Geometry check sheet. Reference: the model listing, model coordinates, mm. A direction names the side the tool comes from. Give positions to 0.01 mm unless a question says otherwise; leave off trailing zeros. Put each result on its own line as item: value. Start each with the question number.
Q1. Material ranges on L1, parallel to Z at x = 76.2, y = 3.5; L2, parallel to X at y = 2, z = -18 (3 decimals); L3, parallel to X at y = 9.5, z = -101 (3 decimals), recorded low to high.
Q2. Section check A-A on y = 8. State how many separate pieces and enclosed holes the cut face has, then the cut area to 3 significant figures.
Q3. Access from +Z, -Z, +X, -X, +Y, -Y to the whole of each face (thin tool, end or side, straight path). Record for faces 4 (the flat face through (46, 6, 0)), 5 (the flat face through (12.7, 6, -16)).
Q4. Mould release check, pull along X, two halves, no side actions. Record for faces 1 (the cylindrical face through (89.359, 6.439, -136.836)), 2 (the flat face through (85.725, 6, -124)), 3 (the cylindrical face through (2.72, 6.44, -136.84)): +X half, -X half, draft (parallel to the pull), parting line (faces both ways), or undercut.
```python
from build123d import *

# Parameters (mm, degrees)
SKETCH1_W                   = 92.075
SKETCH1_H                   = 139.7
BOSS_EXTRUDE1_DEPTH         = 12.7
F_1_4_0_25_DIAMETER_HOLE1_D = 6.35
CUT_EXTRUDE1_DEPTH          = 12.7
FILLET1_R                   = 9.525


with BuildPart() as part:
    # Sketch1 → Boss-Extrude1 (new body)
    with BuildSketch(Plane(origin=(0, 0, 0), x_dir=(1, 0, 0), z_dir=(0, 1, 0))):
        with Locations((46.0375, 69.85)):
            Rectangle(SKETCH1_W, SKETCH1_H)
    extrude(amount=BOSS_EXTRUDE1_DEPTH)

    # 1/4 (0.25) Diameter Hole1 (through all)
    with Locations(Plane(origin=(0, 12.7, 0), x_dir=(1, 0, 0), z_dir=(0, 1, 0))):
        with Locations((76.2, 36.5125), (46.0375, 69.85), (76.2, 103.1875), (15.875, 36.5125), (15.875, 103.1875)):
            Hole(F_1_4_0_25_DIAMETER_HOLE1_D / 2)

    # Sketch7 → Cut-Extrude1 (cut)
    with BuildSketch(Plane(origin=(0, 12.7, 0), x_dir=(1, 0, 0), z_dir=(0, 1, 0))):
        with BuildLine():
            Line((12.7, 127), (12.7, 120.65))
            ThreePointArc((12.7, 120.65), (9.525, 117.475), (6.35, 120.65))
            Line((6.35, 120.65), (6.35, 127))
            ThreePointArc((6.35, 127), (9.525, 130.175), (12.7, 127))
        make_face()
    cut_extrude1 = extrude(amount=-CUT_EXTRUDE1_DEPTH, mode=Mode.SUBTRACT)

    # Sketch-Pattern1: Cut-Extrude1 at 4 more places
    with Locations((36.5125, 0, 53.975), (73.025, 0, 0), (73.025, 0, 107.95), (0, 0, 107.95)):
        add(cut_extrude1, mode=Mode.SUBTRACT)

    # Fillet1
    fillet1_edges = [part.edges().sort_by_distance(p)[0] for p in [
        (0, 6.35, -139.7),
        (92.075, 6.35, -139.7),
        (92.075, 6.35, 0),
        (0, 6.35, 0),
    ]]
    fillet(fillet1_edges, radius=FILLET1_R)


solid = part.part
```
Results found:
1. L1: z = -139.7 to -106.36, -100.01 to -39.69, -33.34 to 0
1. L2: x = 0 to 6.35, 12.7 to 79.375, 85.725 to 92.075
1. L3: x = 0 to 13.574, 18.176 to 73.899, 78.501 to 92.075
2. separate pieces: 1
2. enclosed holes: 9
2. area: 12,300 mm^2
3. face 4: +Z, +X, -X, +Y, -Y
3. face 5: +Y, -Y
4. face 1: +X half
4. face 2: undercut
4. face 3: -X half
